For this review, use the dimensioned drawing (mm, ordinates from the lowest corner) and the shaded views. A direction names the side the tool comes from. Coordinates: 2 decimals unless noted, no trailing zeros. Loops run counter-clockwise (first coordinate to the right, second up) from the corner with the lowest first, then second, coordinate; pieces in that order, holes last. Notation, with made-up numbers: (-36, 79.25) -> (-28, 79.25) arc R21 ccw to (-28, 115.25) -> close; hole circle Ø5 at (37, 26.5). An arc over 180 degrees is marked (long way). Answer as a JSON object with one key per item and string values.
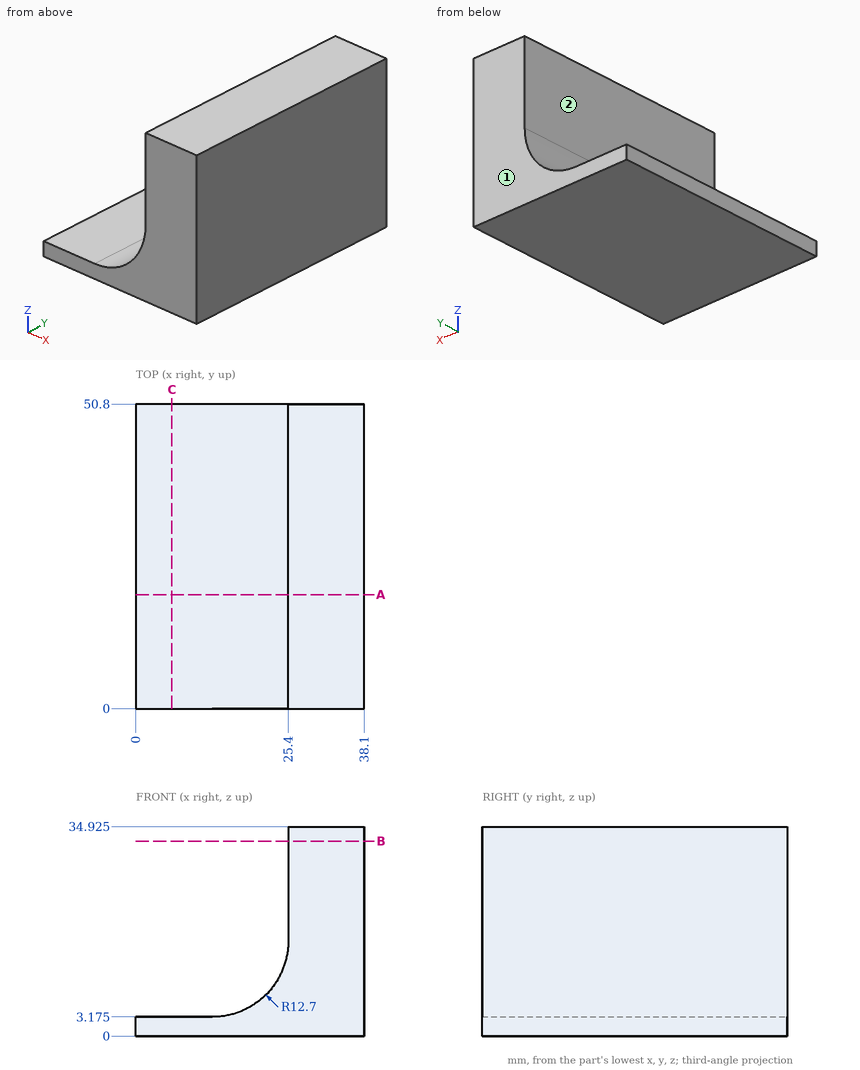
1) Wall thickness on probe 1 along Z at (x, y) = (6, 3) (3 decimals); probe 2 along X at (y, z) = (16, 29.5); probe 3 along Z at (x, y) = (24, 41.5): over which ranges is each line inside the solid? List them lowest first.
Completed:
{"probe 1": "0 to 3.175", "probe 2": "25.4 to 38.1", "probe 3": "0 to 10.08"}
2) Clearance check with flat-ended pins moving along their axes: pin 1 Ø2 at (x, y) = (20, 9) entering from +Z; pin 2 Ø10 at (y, z) = (11.5, 13) entering from -X; pin 3 Ø14 at (x, y) = (4.5, 36) entering from +Z (3 decimals); pin 4 Ø12 at (x, y) = (13.5, 31) entering from -Z. State where each tip first meets the part, or that it passes through.
Completed:
{"pin 1": "z = 6.26", "pin 2": "x = 22.66", "pin 3": "z = 3.175", "pin 4": "z = 0"}
3) Add section B-B, the plane z = 32.5. Give the boundary of the cut face in (x, y).
Completed:
{"outline": "(25.4, 0) -> (38.1, 0) -> (38.1, 50.8) -> (25.4, 50.8) -> close"}
4) For the marked faces 1 and 2, list the 3-axis set-ups (+Z, -Z, +X, -X, +Y, -Y) from which the entire face can be reached by the end or side of a thin tool; tool diameter is ignored.
Completed:
{"face 1": "+Z, -Z, +X, -X, +Y", "face 2": "+Z, -X, +Y, -Y"}
5) Add section A-A, the plane y = 19. Give the boundary of the cut face in (x, z) (3 decimals), and give its area (3 significant figures).
Completed:
{"outline": "(0, 0) -> (38.1, 0) -> (38.1, 34.925) -> (25.4, 34.925) -> (25.4, 15.875) arc R12.7 cw to (12.7, 3.175) -> (0, 3.175) -> close", "area": "559 mm²"}
6) Add section C-C, the plane x = 6. Give the boundary of the cut face in (y, z) (3 decimals).
Completed:
{"outline": "(0, 0) -> (50.8, 0) -> (50.8, 3.175) -> (0, 3.175) -> close"}
